from build123d import *

# Parameters (mm, degrees)
BOSS_EXTRUDE1_DEPTH = 100
SKETCH2_W           = 80
SKETCH2_H           = 80
CUT_EXTRUDE1_DEPTH  = 100
SKETCH3_R           = 40
BOSS_EXTRUDE2_DEPTH = 80


with BuildPart() as part:
    # Sketch1 → Boss-Extrude1 (new body)
    with BuildSketch(Plane(origin=(0, 0, 0), x_dir=(0, 0, -1), z_dir=(1, 0, 0))):
        with BuildLine():
            Line((0, 40), (-80, 40))
            Line((-80, 40), (-80, -40))
            Line((-80, -40), (0, -40))
            ThreePointArc((0, -40), (40, 0), (0, 40))
        make_face()
    extrude(amount=BOSS_EXTRUDE1_DEPTH)

    # Sketch2 → Cut-Extrude1 (cut)
    with BuildSketch(Plane(origin=(0, 40, 0), x_dir=(1, 0, 0), z_dir=(0, 1, 0))):
        with Locations((50, 0)):
            Rectangle(SKETCH2_W, SKETCH2_H)
    extrude(amount=-CUT_EXTRUDE1_DEPTH, mode=Mode.SUBTRACT)

    # Sketch3 → Boss-Extrude2 (add)
    with BuildSketch(Plane.XY.offset(80)):
        with Locations(Location((50, 0, 0), (0, 0, 270))):
            Circle(SKETCH3_R)
    extrude(amount=BOSS_EXTRUDE2_DEPTH)


solid = part.part
Could you check a few things on this model? Use its own coordinates, in mm. A direction names the side the tool comes from. Coordinates: 2 decimals unless noted, no trailing zeros. Order: outer loops, then holes, each group sorted by start corner. A loop starts at its lowest first (then second) coordinate and runs counter-clockwise, first axis right, second up. Notation, with made-up numbers: (39, 67.25) - (56, 67.25) arc R24 cw to (56, 91.25) - close; hole circle Ø1 at (15, 37.5). An arc over 180 degrees is marked (long way). Answer in a Markdown table with one row per item. Add a question column.
(1) If we section it at B-B, the plane x = 74: Please give me the cut outline in (y, z), then the cut area to 3 significant figures.
(2) If we section it at C-C, the plane z = -11.5: Please give me the cut outline in (x, y), then the cut area to 3 significant figures.
(3) I need wall thicknesses on L1, parallel to X at y = -5, z = -9; L2, parallel to Z at x = 86.5, y = -35; L3, parallel to Z at x = 22, y = -13.5. Which ranges of each line are inside material? Lowest first, please.
(4) On a 3-axis mill with a long thin cutter (end or side, diameter ignored), from which of +Z, -Z, +X, -X, +Y, -Y can I reach the whole of each face in a straight line? I mean faces 4 (the face through (0, 1, 21)), 5 (the face through (90, 1, 1)), 6 (the face through (8, 1, 80)). Say none if no direction works.
(5) If we section it at A-A, the plane y = 0: Please give me the cut outline in (x, z).
(6) Will these pins go through, and if not, where does the flat tip stop? pin 1 (1.5 mm diameter, centred on x = 16.5, z = 97, fed in from +Y); pin 2 (5 mm diameter, centred on x = 27, y = 7.5, fed in from -Z); pin 3 (5 mm diameter, centred on y = 6.5, z = 99, fed in from -X).
(7) If we section it at D-D, the plane z = 121: Please give me the cut outline in (x, y).
(8) If we mould it in two halves opening along X, with no side actions, what happens to faces 1 (the face through (10.95, 8.67, 119.44)), 2 (the face through (49, 1, 40)), 3 (the face through (92, 0, 80))? For each: released by +X, released by -X, zero draft, split by the parting line, or undercut.
Results are:
| question | item | result |
|---|---|---|
| 1 | outline | (-40, 40) - (40, 40) - (40, 80) - (32, 80) - (32, 160) - (-32, 160) - (-32, 80) - (-40, 80) - close |
| 1 | area | 8,320 mm2 |
| 2 | outline | (0, -38.31) - (10, -38.31) - (10, 38.31) - (0, 38.31) - close; (90, -38.31) - (100, -38.31) - (100, 38.31) - (90, 38.31) - close |
| 2 | area | 1,530 mm2 |
| 3 | L1 | x = 0 to 10, 90 to 100 |
| 3 | L2 | z = 40 to 80 |
| 3 | L3 | z = 40 to 160 |
| 4 | face 4 | +Z, -Z, -X, +Y, -Y |
| 4 | face 5 | -Z, +Y, -Y |
| 4 | face 6 | +Z, -X |
| 5 | outline | (0, -40) - (10, -40) - (10, 40) - (90, 40) - (90, -40) - (100, -40) - (100, 80) - (90, 80) - (90, 160) - (10, 160) - (10, 80) - (0, 80) - close |
| 6 | pin 1 | stops at y = 22.97 |
| 6 | pin 2 | stops at z = 40 |
| 6 | pin 3 | stops at x = 10.2 |
| 7 | outline | circle Ø80 at (50, 0) |
| 8 | face 1 | split by the parting line |
| 8 | face 2 | undercut |
| 8 | face 3 | zero draft |
